Could you check a few things on this model? Use its own coordinates, in mm. A direction names the side the tool comes from. Round coordinates to 2 decimals unless told otherwise and drop trailing zeros. Write each loop counter-clockwise with the first axis right and the second up, starting at its lowest first coordinate (ties: lowest second). Pieces come first, ordered by that corner, then holes. Notation, with made-up numbers: (7, 38.5) -> (49, 38.5) arc R12 cw to (49, 47.5) -> close; hole circle Ø4 at (2, 12). An arc over 180 degrees is marked (long way). One line per question, with ' | ' between items. Start each with the question number.
1. If I drill on line 1 along X through (y, z) = (7, 0); line 2 along Y through (x, z) = (-0.5, 12); line 3 along Y through (x, z) = (-8.5, -4.25), over which ranges is the centre line in solid material (lowest first)? Write a range as [from, to].
2. For faces 1 (the cylindrical face through (-3.755, 5.972, -11.923)), 2 (the flat face through (-13.899, 1.972, 8.276)), which set-ups out of +Z, -Z, +X, -X, +Y, -Y let a thin tool reach every point of the face, with its end or its side?
3. For pin 1 Ø1.5 at (x, y) = (-16.5, 4.5) entering from -Z; pin 2 Ø1.5 at (y, z) = (7.5, -3) entering from +X; pin 3 Ø3 at (x, z) = (19, 3) entering from +Y, each with a flat end and sliding along its axis, tell me the tip position at first contact or that it passes through.
4. Imagine slicing it at C-C, the plane z = -3.25. List the corners of the cut face in (x, y) for me, and give its area (3 significant figures).
5. Imagine slicing it at B-B, the plane x = 18.25. List the corners of the cut face in (y, z) for me.
6. Imagine slicing it at D-D, the plane y = 10.75. List the corners of the cut face in (x, z) for me, and give its area (3 significant figures).
7. Imagine slicing it at A-A, the plane z = 0. List the corners of the cut face in (x, y) for me, and give its area (3 significant figures).
8. Thinking about a two-plate mould opening in Z: for faces 3 (the cylindrical face through (4.88, 9.2, 1.08)), 4 (the flat face through (-14.1, 1.97, -8.18)), 5 (the flat face through (10, 8, -5)), which applies, released by +Z, released by -Z, zero draft, split by the parting line, or undercut?
from build123d import *

# Parameters (mm, degrees)
BOSS_EXTRUDE1_DEPTH = 4
SKETCH1_3_R         = 12.5
SKETCH1_3_R_2       = 11
BOSS_EXTRUDE2_DEPTH = 8
SKETCH1_4_R         = 5
SKETCH1_4_R_2       = 4
BOSS_EXTRUDE3_DEPTH = 12.5
SKETCH3_R           = 11
SKETCH3_R_2         = 5
BOSS_EXTRUDE4_DEPTH = 2
SKETCH1_5_R         = 4
SKETCH1_5_R_2       = 2.285917385
CUT_EXTRUDE1_DEPTH  = 31.24070105


with BuildPart() as part:
    # Sketch1 → Boss-Extrude1 (new body)
    with BuildSketch(Plane(origin=(0, 0, 0), x_dir=(1, 0, 0), z_dir=(0, 1, 0))):
        with BuildLine():
            Line((-21.25, 4.763139721), (-6.75, 11.691342951))
            ThreePointArc((-6.75, 11.691342951), (0, 13.5), (6.75, 11.691342951))
            Line((6.75, 11.691342951), (21.25, 4.763139721))
            ThreePointArc((21.25, 4.763139721), (24, 0), (21.25, -4.763139721))
            Line((21.25, -4.763139721), (6.75, -11.691342951))
            ThreePointArc((6.75, -11.691342951), (0, -13.5), (-6.75, -11.691342951))
            Line((-6.75, -11.691342951), (-21.25, -4.763139721))
            ThreePointArc((-21.25, -4.763139721), (-24, 0), (-21.25, 4.763139721))
        make_face()
    extrude(amount=BOSS_EXTRUDE1_DEPTH)

    # Sketch1_3 → Boss-Extrude2 (add)
    with BuildSketch(Plane(origin=(0, 0, 0), x_dir=(1, 0, 0), z_dir=(0, 1, 0))):
        with Locations(Location((0, 0, 0), (0, 0, 90))):
            Circle(SKETCH1_3_R)
        with Locations(Location((0, 0, 0), (0, 0, 90))):
            Circle(SKETCH1_3_R_2, mode=Mode.SUBTRACT)
    extrude(amount=BOSS_EXTRUDE2_DEPTH)

    # Sketch1_4 → Boss-Extrude3 (add)
    with BuildSketch(Plane(origin=(0, 0, 0), x_dir=(1, 0, 0), z_dir=(0, 1, 0))):
        with Locations(Location((0, 0, 0), (0, 0, 90))):
            Circle(SKETCH1_4_R)
        with Locations(Location((0, 0, 0), (0, 0, 90))):
            Circle(SKETCH1_4_R_2, mode=Mode.SUBTRACT)
    extrude(amount=BOSS_EXTRUDE3_DEPTH)

    # Sketch3 → Boss-Extrude4 (add)
    with BuildSketch(Plane(origin=(0, 4, 0), x_dir=(1, 0, 0), z_dir=(0, 1, 0))):
        with Locations(Location((0, 0, 0), (0, 0, 270))):
            Circle(SKETCH3_R)
        with Locations(Location((0, 0, 0), (0, 0, 270))):
            Circle(SKETCH3_R_2, mode=Mode.SUBTRACT)
    extrude(amount=BOSS_EXTRUDE4_DEPTH)

    # Sketch1_5 → Cut-Extrude1 (cut, through all)
    with BuildSketch(Plane(origin=(0, 0, 0), x_dir=(1, 0, 0), z_dir=(0, 1, 0))):
        with Locations(Location((0, 0, 0), (0, 0, 270))):
            Circle(SKETCH1_5_R)
        with Locations(Location((18.25, 0, 0), (0, 0, 90))):
            Circle(SKETCH1_5_R_2)
        with Locations(Location((-18.25, 0, 0), (0, 0, 90))):
            Circle(SKETCH1_5_R_2)
    extrude(amount=CUT_EXTRUDE1_DEPTH, mode=Mode.SUBTRACT)


solid = part.part
Geometry results:
1) line 1: x = [-12.5, -11], [-5, -4], [4, 5], [11, 12.5] | line 2: y = [0, 8] | line 3: y = [0, 6]
2) face 1: +Y | face 2: +Z, -X, +Y, -Y
3) pin 1: stops at z = -7.3 | pin 2: stops at x = 12.3 | pin 3: stops at y = 4
4) outline: (-22.94, 0) -> (-2.33, 0) -> (-2.33, 12.5) -> (-3.8, 12.5) -> (-3.8, 6) -> (-10.51, 6) -> (-10.51, 8) -> (-12.07, 8) -> (-12.07, 4) -> (-22.94, 4) -> close; (2.33, 0) -> (22.94, 0) -> (22.94, 4) -> (12.07, 4) -> (12.07, 8) -> (10.51, 8) -> (10.51, 6) -> (3.8, 6) -> (3.8, 12.5) -> (2.33, 12.5) -> close | area: 229 mm2
5) outline: (0, -6.2) -> (4, -6.2) -> (4, -2.29) -> (0, -2.29) -> close; (0, 2.29) -> (4, 2.29) -> (4, 6.2) -> (0, 6.2) -> close
6) outline: circle Ø10 at (0, 0); hole circle Ø8 at (0, 0) | area: 28.3 mm2
7) outline: (-24, 0) -> (-20.54, 0) -> (-20.54, 4) -> (-24, 4) -> close; (-15.96, 0) -> (-4, 0) -> (-4, 12.5) -> (-5, 12.5) -> (-5, 6) -> (-11, 6) -> (-11, 8) -> (-12.5, 8) -> (-12.5, 4) -> (-15.96, 4) -> close; (4, 0) -> (15.96, 0) -> (15.96, 4) -> (12.5, 4) -> (12.5, 8) -> (11, 8) -> (11, 6) -> (5, 6) -> (5, 12.5) -> (4, 12.5) -> close; (20.54, 0) -> (24, 0) -> (24, 4) -> (20.54, 4) -> close | area: 176 mm2
8) face 3: undercut | face 4: released by -Z | face 5: zero draft
